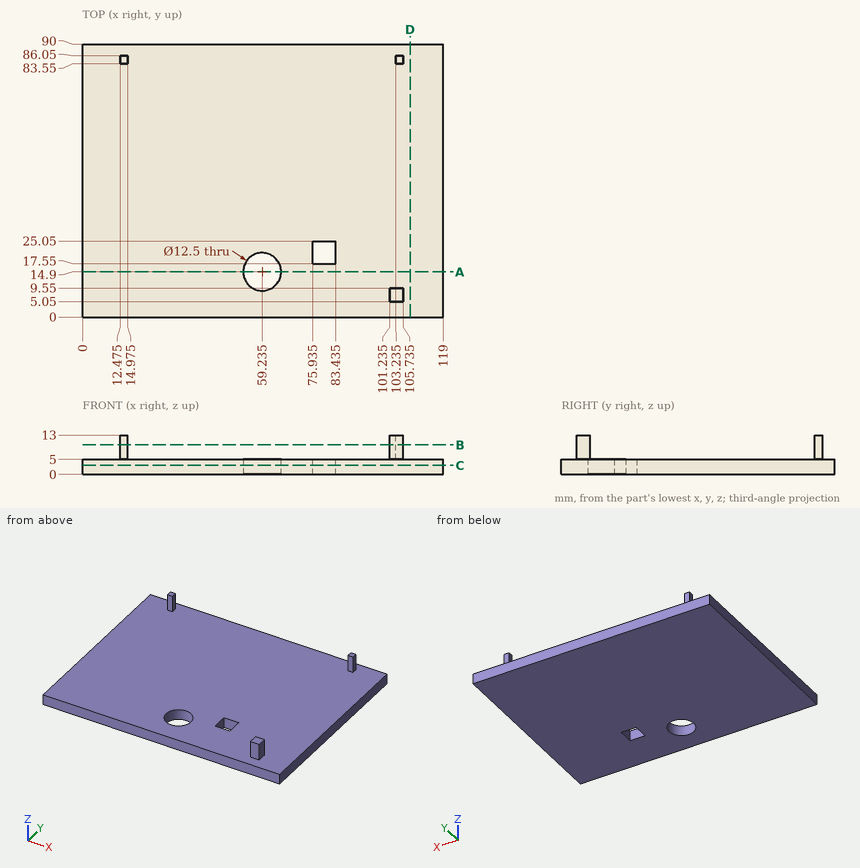
Verification items for this drawing (mm, ordinates from the low corner). Give positions to 0.01 mm unless a question says otherwise; leave off trailing zeros. Loops run counter-clockwise (first coordinate to the right, second up) from the corner with the lowest first, then second, coordinate; pieces in that order, holes last. Notation, with made-up numbers: M -38.5,-22.5 L -14.5,-22.5 A25 ccw -14.5,-5.5 Z; hole C 43,64.25 d10. An arc over 180 degrees is marked long. Answer in a Markdown table with one row per item.
1) Cross-section at D-D (x = 108). Enter the section's corners in (y, z), plus the area to 3 significant figures.
Solutions:
| item | result |
|---|---|
| outline | M 0,0 L 90,0 L 90,5 L 0,5 Z |
| area | 450 mm^2 |
2) Cross-section at A-A (y = 14.9). Enter the section's corners in (x, z) (3 decimals), plus the area to 4 significant figures.
Solutions:
| item | result |
|---|---|
| outline | M 0,0 L 52.985,0 L 52.985,5 L 0,5 Z; M 65.485,0 L 119,0 L 119,5 L 65.485,5 Z |
| area | 532.5 mm^2 |
3) Cross-section at C-C (z = 3). Enter the section's corners in (x, y) (3 decimals), plus the area to 3 significant figures.
Solutions:
| item | result |
|---|---|
| outline | M 0,0 L 119,0 L 119,90 L 0,90 Z; hole C 59.235,14.9 d12.5; hole M 75.935,17.55 L 83.435,17.55 L 83.435,25.05 L 75.935,25.05 Z |
| area | 10,500 mm^2 |
4) Cross-section at B-B (z = 9.75). Enter the section's corners in (x, y) (3 decimals), plus the area to 4 significant figures.
Solutions:
| item | result |
|---|---|
| outline | M 12.475,83.55 L 14.975,83.55 L 14.975,86.05 L 12.475,86.05 Z; M 101.235,5.05 L 105.735,5.05 L 105.735,9.55 L 101.235,9.55 Z; M 103.235,83.55 L 105.735,83.55 L 105.735,86.05 L 103.235,86.05 Z |
| area | 32.75 mm^2 |
5) Depth check by flat-ended pin: pin 1 (3 mm diameter, centred on x = 13.5, z = 7, fed in from +Y); pin 2 (8 mm diameter, centred on x = 67.5, y = 63, fed in from +Z); pin 3 (1.5 mm diameter, centred on y = 23, z = 2.5, fed in from -X); pin 4 (3 mm diameter, centred on x = 105, z = 8.5, fed in from -Y). Enter the tip coordinate at first touch or a pass-through.
Solutions:
| item | result |
|---|---|
| pin 1 | stops at y = 86.05 |
| pin 2 | stops at z = 5 |
| pin 3 | stops at x = 0 |
| pin 4 | stops at y = 5.05 |
6) Thickness scan on line 1 (Y direction, x = 80, z = 3); line 2 (Z direction, x = 108, y = 29). Record the ranges inside material, lowest first.
Solutions:
| item | result |
|---|---|
| line 1 | y = 0 to 17.55, 25.05 to 90 |
| line 2 | z = 0 to 5 |
